from build123d import *

# Parameters (mm, degrees)
ESBO_O1_W                = 107
ESBO_O1_H                = 22.62
RESSALTO_EXTRUS_O1_DEPTH = 3.5
ESBO_O1_4_R              = 3.5
RESSALTO_EXTRUS_O2_DEPTH = 5.5
ESBO_O1_7_R              = 1.5
CORTE_EXTRUS_O1_DEPTH    = 5.5
ESBO_O1_9_R              = 1.5
RESSALTO_EXTRUS_O4_DEPTH = 3.5


with BuildPart() as part:
    # Esboço1 → Ressalto-extrusão1 (new body)
    with BuildSketch(Plane.XY):
        with Locations((12.82231405, 21.961694215)):
            Rectangle(ESBO_O1_W, ESBO_O1_H)
    extrude(amount=RESSALTO_EXTRUS_O1_DEPTH)

    # Esboço1<4> → Ressalto-extrusão2 (add)
    with BuildSketch(Plane.XY):
        with Locations((14.32231405, 17.551694215)):
            Circle(ESBO_O1_4_R)
        with Locations((32.32231405, 17.551694215)):
            Circle(ESBO_O1_4_R)
        with Locations((50.32231405, 17.551694215)):
            Circle(ESBO_O1_4_R)
    extrude(amount=RESSALTO_EXTRUS_O2_DEPTH)

    # Esboço1<7> → Corte-extrusão1 (cut)
    with BuildSketch(Plane.XY):
        with Locations((14.32231405, 17.551694215)):
            Circle(ESBO_O1_7_R)
        with Locations((32.32231405, 17.551694215)):
            Circle(ESBO_O1_7_R)
        with Locations((50.32231405, 17.551694215)):
            Circle(ESBO_O1_7_R)
    extrude(amount=CORTE_EXTRUS_O1_DEPTH, mode=Mode.SUBTRACT)

    # Esboço1<9> → Ressalto-extrusão4 (add)
    with BuildSketch(Plane.XY):
        with Locations((14.32231405, 17.551694215)):
            Circle(ESBO_O1_9_R)
        with Locations((32.32231405, 17.551694215)):
            Circle(ESBO_O1_9_R)
        with Locations((50.32231405, 17.551694215)):
            Circle(ESBO_O1_9_R)
    extrude(amount=RESSALTO_EXTRUS_O4_DEPTH)


solid = part.part
Verification items for the finished model (mm, model axes). A direction names the side the tool comes from. Coordinates: 2 decimals unless noted, no trailing zeros. Order: outer loops, then holes, each group sorted by start corner. A loop starts at its lowest first (then second) coordinate and runs counter-clockwise, first axis right, second up. Notation, with made-up numbers: M 82.25,29 L 119.25,29 A22 ccw 119.25,52 Z; hole C 54,-1 d3. An arc over 180 degrees is marked long. One line per item, written item: value. Start each with the question number.
Item 1: Sectioned sample at A-A (z = 4.35). Enter the section's corners in (x, y), then the cut area to 3 significant figures.
Item 2: Mould release check, pull along Y, two halves, no side actions. Record for faces 1 (the cylindrical face through (53.66, 18.6, 4.49)), 2 (the flat face through (14, 18, 3.5)), 3 (the flat face through (34, 18, 5.5)): released by +Y, released by -Y, zero draft, split by the parting line, or undercut.
Item 3: Sectioned sample at C-C (y = 24.5). Enter the section's corners in (x, z), then the cut area to 4 significant figures.
Item 4: Access from +Z, -Z, +X, -X, +Y, -Y to the whole of each face (thin tool, end or side, straight path). Record for faces 4 (the flat face through (12, 10.652, 2)), 5 (the cylindrical face through (29.743, 19.917, 4.486)).
Item 5: Gauge pin test, flat end, axial feed: pin 1 (1.5 mm diameter, centred on x = 32, y = 17.5, fed in from +Z). Record the tip position at first contact, or that the pin passes through.
Item 6: Sectioned sample at B-B (x = -30.5). Enter the section's corners in (y, z), then the cut area to 3 significant figures.
Item 7: Scan lines: probe 1 along X at (y, z) = (20, 4.25); probe 2 along Z at (x, y) = (-19, 17); probe 3 along Y at (x, z) = (12, 4.75). Record each from-to range of solid material in increasing order.
Conclusion:
1. outline: C 14.32,17.55 d7; C 32.32,17.55 d7; C 50.32,17.55 d7; hole C 14.32,17.55 d3; hole C 32.32,17.55 d3; hole C 50.32,17.55 d3
1. area: 94.2 mm^2
2. face 1: split by the parting line
2. face 2: undercut
2. face 3: zero draft
3. outline: M -40.68,0 L 66.32,0 L 66.32,3.5 L -40.68,3.5 Z
3. area: 374.5 mm^2
4. face 4: +Z, -Z, +X, -X, -Y
4. face 5: +Z
5. pin 1: stops at z = 3.5
6. outline: M 10.65,0 L 33.27,0 L 33.27,3.5 L 10.65,3.5 Z
6. area: 79.2 mm^2
7. probe 1: x = 11.82 to 16.82, 29.82 to 34.82, 47.82 to 52.82
7. probe 2: z = 0 to 3.5
7. probe 3: y = 14.93 to 20.17
